```python
from build123d import *

# Parameters (mm, degrees)
BOSS_EXTRUDE1_DEPTH                           = 9.5
CBORE_FOR_M12_HEX_HEAD_CAP_SCREW1_D           = 6.75
CBORE_FOR_M12_HEX_HEAD_CAP_SCREW1_DEPTH       = 16.51
CBORE_FOR_M12_HEX_HEAD_CAP_SCREW1_CBORE_D     = 25
CBORE_FOR_M12_HEX_HEAD_CAP_SCREW1_CBORE_DEPTH = 5


with BuildPart() as part:
    # Sketch1 → Boss-Extrude1 (new, symmetric)
    with BuildSketch(Plane(origin=(0, 0, 0), x_dir=(0, 0, -1), z_dir=(1, 0, 0))):
        with BuildLine():
            Line((12.7, 0), (25.4, 0))
            Line((25.4, 0), (25.4, 19))
            Line((25.4, 19), (-25.4, 19))
            Line((-25.4, 19), (-25.4, 0))
            Line((-25.4, 0), (-12.7, 0))
            ThreePointArc((-12.7, 0), (0, 12.7), (12.7, 0))
        make_face()
    extrude(amount=BOSS_EXTRUDE1_DEPTH, both=True)

    # CBORE for M12 Hex Head Cap Screw1
    with Locations(Plane(origin=(0, 19, 0), x_dir=(1, 0, 0), z_dir=(0, 1, 0))):
        with Locations((0, 19.05), (0, -19.05)):
            CounterBoreHole(CBORE_FOR_M12_HEX_HEAD_CAP_SCREW1_D / 2, CBORE_FOR_M12_HEX_HEAD_CAP_SCREW1_CBORE_D / 2, CBORE_FOR_M12_HEX_HEAD_CAP_SCREW1_CBORE_DEPTH, depth=CBORE_FOR_M12_HEX_HEAD_CAP_SCREW1_DEPTH)


solid = part.part
```
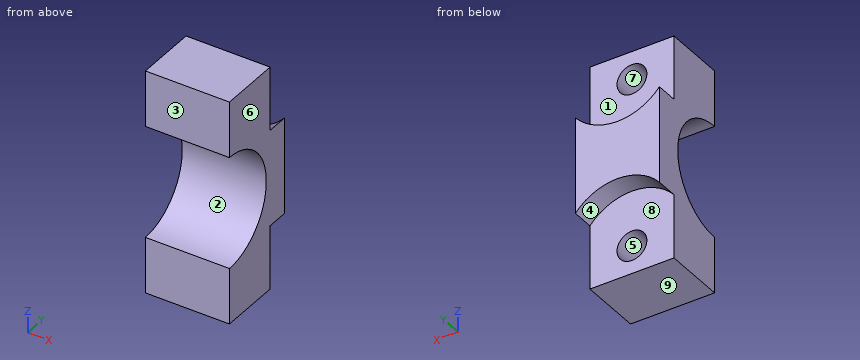
Part model, mm, in its own coordinate system. Face numbers are marked on the shaded views. A direction names the side the tool comes from. Round coordinates to 2 decimals unless told otherwise and drop trailing zeros. Loops run counter-clockwise (first coordinate to the right, second up) from the corner with the lowest first, then second, coordinate; pieces in that order, holes last.
1. Flat gauge pins, fed straight in: pin 1 (1.5 mm diameter, centred on x = 1, z = -6.5, fed in from -Y); pin 2 (3.5 mm diameter, centred on x = -0.5, z = 18.5, fed in from +Y); pin 3 (9.5 mm diameter, centred on x = 3, z = -20.5, fed in from +Y); pin 4 (10 mm diameter, centred on x = -2.5, y = 15.5, fed in from -Z). Where does each tip first touch, or does it go through?
Solutions:
pin 1: stops at y = 10.43
pin 2: stops at y = 2.49
pin 3: stops at y = 14
pin 4: stops at z = -25.4
2. 3-axis set-ups, long thin cutter, end or side, ignore diameter. For the marked faces 1, 2, 3, 4 and 5: which of +Z, -Z, +X, -X, +Y, -Y reach the whole face in a straight line?
Solutions:
face 1: +Z, +Y
face 2: +X, -X, -Y
face 3: +Z, -Z, +X, -X, -Y
face 4: -Z, +Y
face 5: +Y
3. Slice it at D-D (y = 9.5). Give the cut face in (x, z) (3 decimals).
Solutions:
outline: (-9.5, -25.4) - (9.5, -25.4) - (9.5, -8.429) - (-9.5, -8.429) - close; (-9.5, 8.429) - (9.5, 8.429) - (9.5, 25.4) - (-9.5, 25.4) - close; hole circle Ø6.75 at (0, -19.05); hole circle Ø6.75 at (0, 19.05)
4. Slice it at A-A (y = 6.75). Give the cut face in (x, z) (3 decimals), and give its area (3 significant figures).
Solutions:
outline: (-9.5, -25.4) - (9.5, -25.4) - (9.5, -10.758) - (-9.5, -10.758) - close; (-9.5, 10.758) - (9.5, 10.758) - (9.5, 25.4) - (-9.5, 25.4) - close; hole circle Ø6.75 at (0, -19.05); hole circle Ø6.75 at (0, 19.05)
area: 485 mm2
5. Slice it at C-C (x = 5). Give the cut face in (y, z).
Solutions:
outline: (0, -25.4) - (14, -25.4) - (14, -7.59) - (19, -7.59) - (19, 7.59) - (14, 7.59) - (14, 25.4) - (0, 25.4) - (0, 12.7) arc R12.7 cw to (0, -12.7) - close
6. Drill centre lines: line 1 along X through (y, z) = (7.5, -19.05) (3 decimals); line 2 along Z through (x, y) = (0, 8.25) (3 decimals); line 3 along Z through (x, y) = (0.25, 8). Where is each one in solid material? Low to high.
Solutions:
line 1: x = -9.5 to -3.375, 3.375 to 9.5
line 2: z = -25.4 to -22.425, -15.675 to -9.655, 9.655 to 15.675, 22.425 to 25.4
line 3: z = -25.4 to -22.42, -15.68 to -9.86, 9.86 to 15.68, 22.42 to 25.4
7. Slice it at B-B (z = -19.05). Give the cut face in (x, y) (3 decimals).
Solutions:
outline: (-9.5, 0) - (9.5, 0) - (9.5, 14) - (3.375, 14) - (3.375, 2.49) - (-3.375, 2.49) - (-3.375, 14) - (-9.5, 14) - close
8. Two-plate mould, pull along X, no slides. Class the marked faces 6, 7, 8 and 9: pulls with the +X half, pulls with the -X half, needs draft (parallel to the pull), parting line crosses it, or undercut.
Solutions:
face 6: pulls with the +X half
face 7: undercut
face 8: undercut
face 9: needs draft
